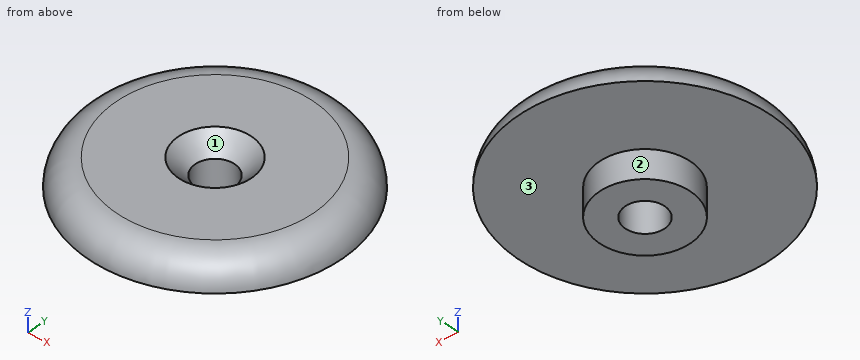
```python
from build123d import *

# Parameters (mm, degrees)
F0_R           = 11.25
F1_DEPTH       = 2.5
F2_R           = 2.49999
F4_R           = 4.05
F5_DEPTH       = 2.5
F6_D           = 3.5
F6_DEPTH       = 7
F6_CSINK_D     = 6.5
F6_CSINK_ANGLE = 90
F6_TIP         = 1.0515060833


# Not quite as in the source:
# - a fillet or chamfer is up to 0.001 mm smaller than in the source, because OpenCascade refuses the exact size


with BuildPart() as f1:
    # F0 (on Top) → F1 (new body)
    with BuildSketch(Plane.XY):
        Circle(F0_R)
    extrude(amount=F1_DEPTH)

    # F2 (radius 2.5 in the source; OpenCascade refuses exactly that, so slightly less here)
    f2_edges = [f1.edges().sort_by_distance(p)[0] for p in [
        (-11.25, 0, 2.5),
    ]]
    fillet(f2_edges, radius=F2_R)

    # F4 (on face) → F5 (join)
    with BuildSketch(Plane(origin=(0, 0, 0), x_dir=(1, 0, 0), z_dir=(0, 0, -1))):
        Circle(F4_R)
    extrude(amount=F5_DEPTH)

    # F6
    with Locations(Plane.XY.offset(2.5)):
        with Locations((0, 0)):
            CounterSinkHole(F6_D / 2, F6_CSINK_D / 2, depth=F6_DEPTH, counter_sink_angle=F6_CSINK_ANGLE)
            with Locations((0, 0, -(F6_DEPTH + F6_TIP / 2))):  # 118° drill point
                Cone(0, F6_D / 2, F6_TIP, mode=Mode.SUBTRACT)


solid = f1.part
```
Part model, mm, in its own coordinate system. Face numbers are marked on the shaded views. Round coordinates to 2 decimals unless told otherwise and drop trailing zeros. Order: outer loops, then holes, each group sorted by start corner. A loop starts at its lowest first (then second) coordinate and runs counter-clockwise, first axis right, second up. Notation, with made-up numbers: M 78.25,-5.5 L 126.25,-5.5 A7 ccw 126.25,-1.5 Z; hole C 19.5,2.25 d7. An arc over 180 degrees is marked long. Answer in a Markdown table with one row per item. Add a question column.
Q1. Cut at D-D on z = 1.8. Give the cut face in (x, y).
Q2. Cut at C-C on z = -1.55. Give the cut face in (x, y), and give its area (3 significant figures).
Q3. Wall check: L1, parallel to Y at x = 0, z = -0.55; L2, parallel to Z at x = -5, y = -4.75. Give the ranges that are in metal, low to high. Write a range as from..to.
Q4. Pin check, flat tips, straight feed: pin 1 (2 mm diameter, centred on y = 3.5, z = 2, fed in from -X); pin 2 (3 mm diameter, centred on x = 1.5, z = -1, fed in from +Y); pin 3 (8 mm diameter, centred on x = -8, y = -8.5, fed in from -Z). Stop position of each tip, or through.
Q5. Mould opens along X. For the marked faces 1, 2 and 3 say: +X half, -X half, draft (parallel to the pull), parting line (faces both ways), or undercut.
Established:
| question | item | result |
|---|---|---|
| 1 | outline | C 0,0 d20.97; hole C 0,0 d5.1 |
| 2 | outline | C 0,0 d8.1; hole C 0,0 d3.5 |
| 2 | area | 41.9 mm2 |
| 3 | L1 | y = -4.05..-1.75, 1.75..4.05 |
| 3 | L2 | z = 0..2.5 |
| 4 | pin 1 | stops at x = -10.56 |
| 4 | pin 2 | stops at y = 11.24 |
| 4 | pin 3 | stops at z = 0 |
| 5 | face 1 | undercut |
| 5 | face 2 | parting line |
| 5 | face 3 | draft |
